```python
from build123d import *

# Parameters (mm, degrees)
F0_W     = 108.3868816495
F0_H     = 72.5326761603
F1_DEPTH = 25
F3_D     = 4.1
F3_DEPTH = 10
F3_TIP   = 1.231764269
F4_D     = 5.5
F4_DEPTH = 10
F4_TIP   = 1.6523667023
F5_D     = 5
F5_DEPTH = 10
F5_TIP   = 1.5021515476


with BuildPart() as f1:
    # F0 (on Top) → F1 (new body)
    with BuildSketch(Plane.XY):
        Rectangle(F0_W, F0_H)
    extrude(amount=F1_DEPTH)

    # F3
    with Locations(Plane.XY.offset(25)):
        with Locations((-43.7879338861, 0)):
            Hole(F3_D / 2, depth=F3_DEPTH)
            with Locations((0, 0, -(F3_DEPTH + F3_TIP / 2))):  # 118° drill point
                Cone(0, F3_D / 2, F3_TIP, mode=Mode.SUBTRACT)

    # F4
    with Locations(Plane.XY.offset(25)):
        with Locations((-23.7893629819, 0)):
            Hole(F4_D / 2, depth=F4_DEPTH)
            with Locations((0, 0, -(F4_DEPTH + F4_TIP / 2))):  # 118° drill point
                Cone(0, F4_D / 2, F4_TIP, mode=Mode.SUBTRACT)

    # F5
    with Locations(Plane.XY.offset(25)):
        with Locations((-8.0840988085, 0)):
            Hole(F5_D / 2, depth=F5_DEPTH)
            with Locations((0, 0, -(F5_DEPTH + F5_TIP / 2))):  # 118° drill point
                Cone(0, F5_D / 2, F5_TIP, mode=Mode.SUBTRACT)


solid = f1.part
```
Design review of the part built by this model. Coordinates are the model's own, in mm. A direction names the side the tool comes from. Give positions to 0.01 mm unless a question says otherwise; leave off trailing zeros. Return JSON: item names as keys, results as strings. Group by question number.
Item 1: Mouldability with a two-part tool opening along X and no side actions: class faces 1 (the cylindrical face through (-21.04, 0.12, 19.93)), 2 (the conical face through (-23.348, -0.183, 13.635)), 3 (the flat face through (-54.193, -1, 12)), 4 (the flat face through (-1, 1, 0)) as released by +X, released by -X, zero draft, split by the parting line, or undercut.
Item 2: Insertion check: pin 1 Ø3.5 at (x, y) = (-43.79, 0) entering from +Z. The pin has a flat end and moves straight along its axis. Give the tip position at first contact, or say it passes through.
Item 3: For probe 1 along X at (y, z) = (0, 21.75); probe 2 along Y at (x, z) = (-45.5, 19.25); probe 3 along Y at (x, z) = (-21.5, 17.25), list the stretches that pass through material, from the lowest coordinate up.
Item 4: Tool access review of faces 5 (the cylindrical face through (-10.47, 0.75, 19.93)), 6 (the flat face through (-1, 36.266, 12)): name each direction out of +Z, -Z, +X, -X, +Y, -Y from which nothing blocks a thin tool from reaching the whole face with its end or side.
Output:
{
 "1": {"face 1": "undercut", "face 2": "undercut", "face 3": "released by -X", "face 4": "zero draft"},
 "2": {"pin 1": "stops at z = 14.82"},
 "3": {"probe 1": "x = -54.19 to -45.84, -41.74 to -26.54, -21.04 to -10.58, -5.58 to 54.19", "probe 2": "y = -36.27 to -1.13, 1.13 to 36.27", "probe 3": "y = -36.27 to -1.52, 1.52 to 36.27"},
 "4": {"face 5": "+Z", "face 6": "+Z, -Z, +X, -X, +Y"}
}
